Geometry: final body of the model. Coordinates: model frame, mm. A direction names the side the tool comes from. Coordinates: 2 decimals unless noted, no trailing zeros. Order: outer loops, then holes, each group sorted by start corner. A loop starts at its lowest first (then second) coordinate and runs counter-clockwise, first axis right, second up. Notation, with made-up numbers: (42.25, 76.25) -> (61.25, 76.25) arc R10 cw to (61.25, 80.25) -> close; hole circle Ø5 at (-1.75, -14.75). An arc over 180 degrees is marked (long way). Answer in a Markdown table with one row per item. Add a question column.
1) Pull-direction query (Y, two-part tool) for faces 1 (the face through (15.6, 2.5, 10.5)), 2 (the face through (23, 10, 8)), 3 (the face through (33, 2.5, 10)); classes: +Y half, -Y half, draft (parallel to the pull), parting line (faces both ways), or undercut.
2) Contact query for flat-ended pins moving along their axis: P1, Ø1.2, axis at y = 6.5, z = 10, coming from the +X side; P2, Ø1.2, axis at x = 17, z = 10, coming from the +Y side; P3, Ø0.8, axis at y = 6.5, z = 10.5, coming from the +X side. Output: stop coordinate, or through.
3) Section query D-D on x = 41.5. Return the cut outline in (y, z).
4) Ray query, line 1 (Y direction, x = 41.5, z = 0.55); line 2 (Y direction, x = 29, z = -8.75); line 3 (Y direction, x = 31, z = 4.75). Return the intervals inside material, ascending. Write a range as from..to.
5) Section query C-C on y = 20.5. Return the cut outline in (x, z).
6) Set-up query: faces 4 (the face through (29.425, 6, 10)), 5 (the face through (23, 2, 8)), 6 (the face through (33.4, 9.25, 10.5)), 7 (the face through (37.425, 6, 10)), 8 (the face through (33.5, 28, -6)). Return all of +Z, -Z, +X, -X, +Y, -Y with unobstructed straight access to the full face (end or side cutting, diameter ignored); none if empty.
7) Section query A-A on y = 28. Return the cut outline in (x, z).
8) Section query B-B on x = 17.5. Return the cut outline in (y, z), then the cut area to 3 significant figures.
```python
from build123d import *

# Parameters (mm, degrees)
SKETCH2_W           = 46
SKETCH2_H           = 38
SKETCH2_R           = 1.5
BOSS_EXTRUDE1_DEPTH = 1.5
SKETCH3_W           = 30
SKETCH3_H           = 12
BOSS_EXTRUDE2_DEPTH = 6.5
SKETCH4_W           = 30
SKETCH4_H           = 8
BOSS_EXTRUDE3_DEPTH = 9.5
SKETCH5_W           = 15
SKETCH5_H           = 7.5
BOSS_EXTRUDE4_DEPTH = 11
SKETCH6_W           = 14.5
SKETCH6_H           = 7
CUT_EXTRUDE1_DEPTH  = 11
SKETCH9_W           = 8
SKETCH9_H           = 7
BOSS_EXTRUDE5_DEPTH = 11
SKETCH10_W          = 7.5
SKETCH10_H          = 6.5
CUT_EXTRUDE2_DEPTH  = 11
SKETCH12_W          = 21
SKETCH12_H          = 20
BOSS_EXTRUDE6_DEPTH = 12
SKETCH13_W          = 18
SKETCH13_H          = 12
BOSS_EXTRUDE7_DEPTH = 2


with BuildPart() as part:
    # Sketch2 → Boss-Extrude1 (new body)
    with BuildSketch(Plane.XY):
        with Locations((23, 19)):
            Rectangle(SKETCH2_W, SKETCH2_H)
        with Locations((4.5, 28)):
            Circle(SKETCH2_R, mode=Mode.SUBTRACT)
        with Locations((4.5, 5.5)):
            Circle(SKETCH2_R, mode=Mode.SUBTRACT)
        with Locations((41.5, 5.5)):
            Circle(SKETCH2_R, mode=Mode.SUBTRACT)
        with Locations((41.5, 28)):
            Circle(SKETCH2_R, mode=Mode.SUBTRACT)
    extrude(amount=BOSS_EXTRUDE1_DEPTH)

    # Sketch3 → Boss-Extrude2 (add)
    with BuildSketch(Plane.XY):
        with Locations((23, 6)):
            Rectangle(SKETCH3_W, SKETCH3_H)
    extrude(amount=BOSS_EXTRUDE2_DEPTH)

    # Sketch4 → Boss-Extrude3 (add)
    with BuildSketch(Plane.XY):
        with Locations((23, 6)):
            Rectangle(SKETCH4_W, SKETCH4_H)
    extrude(amount=BOSS_EXTRUDE3_DEPTH)

    # Sketch5 → Boss-Extrude4 (add)
    with BuildSketch(Plane.XY):
        with Locations((15.75, 6)):
            Rectangle(SKETCH5_W, SKETCH5_H)
    extrude(amount=BOSS_EXTRUDE4_DEPTH)

    # Sketch6 → Cut-Extrude1 (cut)
    with BuildSketch(Plane.XY.offset(10)):
        with Locations((15.75, 6)):
            Rectangle(SKETCH6_W, SKETCH6_H)
    extrude(amount=CUT_EXTRUDE1_DEPTH, mode=Mode.SUBTRACT)

    # Sketch9 → Boss-Extrude5 (add)
    with BuildSketch(Plane.XY):
        with Locations((33.424570799, 6)):
            Rectangle(SKETCH9_W, SKETCH9_H)
    extrude(amount=BOSS_EXTRUDE5_DEPTH)

    # Sketch10 → Cut-Extrude2 (cut)
    with BuildSketch(Plane.XY.offset(10)):
        with Locations((33.424570799, 6)):
            Rectangle(SKETCH10_W, SKETCH10_H)
    extrude(amount=CUT_EXTRUDE2_DEPTH, mode=Mode.SUBTRACT)

    # Sketch12 → Boss-Extrude6 (add)
    with BuildSketch(Plane.XY):
        with Locations((23, 28)):
            Rectangle(SKETCH12_W, SKETCH12_H)
    extrude(amount=-BOSS_EXTRUDE6_DEPTH)

    # Sketch13 → Boss-Extrude7 (add)
    with BuildSketch(Plane.XY):
        with Locations((23, 27.789125994)):
            Rectangle(SKETCH13_W, SKETCH13_H)
    extrude(amount=BOSS_EXTRUDE7_DEPTH)


solid = part.part
```
Result:
| question | item | result |
|---|---|---|
| 1 | face 1 | undercut |
| 1 | face 2 | +Y half |
| 1 | face 3 | -Y half |
| 2 | P1 | x = 38 |
| 2 | P2 | y = 10 |
| 2 | P3 | x = 37.42 |
| 3 | outline | (0, 0) -> (4, 0) -> (4, 1.5) -> (0, 1.5) -> close; (7, 0) -> (26.5, 0) -> (26.5, 1.5) -> (7, 1.5) -> close; (29.5, 0) -> (38, 0) -> (38, 1.5) -> (29.5, 1.5) -> close |
| 4 | line 1 | 0..4, 7..26.5, 29.5..38 |
| 4 | line 2 | 18..38 |
| 4 | line 3 | 0..12 |
| 5 | outline | (0, 0) -> (12.5, 0) -> (12.5, -12) -> (33.5, -12) -> (33.5, 0) -> (46, 0) -> (46, 1.5) -> (0, 1.5) -> close |
| 6 | face 4 | +Z, +Y, -Y |
| 6 | face 5 | +Z, +X, -X, -Y |
| 6 | face 6 | +Z |
| 6 | face 7 | +Z, +X, +Y, -Y |
| 6 | face 8 | -Z, +X, +Y, -Y |
| 7 | outline | (0, 0) -> (3, 0) -> (3, 1.5) -> (0, 1.5) -> close; (6, 0) -> (12.5, 0) -> (12.5, -12) -> (33.5, -12) -> (33.5, 0) -> (40, 0) -> (40, 1.5) -> (32, 1.5) -> (32, 2) -> (14, 2) -> (14, 1.5) -> (6, 1.5) -> close; (43, 0) -> (46, 0) -> (46, 1.5) -> (43, 1.5) -> close |
| 8 | outline | (0, 0) -> (18, 0) -> (18, -12) -> (38, -12) -> (38, 1.5) -> (33.79, 1.5) -> (33.79, 2) -> (21.79, 2) -> (21.79, 1.5) -> (12, 1.5) -> (12, 6.5) -> (10, 6.5) -> (10, 9.5) -> (9.75, 9.5) -> (9.75, 11) -> (9.5, 11) -> (9.5, 10) -> (2.5, 10) -> (2.5, 11) -> (2.25, 11) -> (2.25, 9.5) -> (2, 9.5) -> (2, 6.5) -> (0, 6.5) -> close |
| 8 | area | 391 mm2 |
